from build123d import *

# Parameters (mm, degrees)
SKETCH1_R                 = 10.275
SKETCH1_R_2               = 8.275
BOSS_EXTRUDE3_DEPTH       = 5
SKETCH1_6_R               = 8.275
SKETCH1_6_R_2             = 6.025
BOSS_EXTRUDE4_DEPTH       = 18
BOSS_EXTRUDE7_DEPTH       = 40
BOSS_EXTRUDE7_DEPTH_BACK  = 70
SKETCH4_R                 = 25
SKETCH4_R_2               = 23
SKETCH7_W                 = 197.712308018
SKETCH7_H                 = 113.854833504
CUT_EXTRUDE4_DEPTH        = 64
BOSS_EXTRUDE9_START       = -2
SKETCH9_RX                = 35.355339059
SKETCH9_RY                = 25
SKETCH9_R                 = 6.025
BOSS_EXTRUDE9_DEPTH       = 2
BOSS_EXTRUDE12_DEPTH      = 2
BOSS_EXTRUDE12_DEPTH_BACK = 4
SKETCH22_W                = 69.752550136
SKETCH22_H                = 19.780641822
CUT_EXTRUDE5_DEPTH        = 10
BOSS_EXTRUDE13_START      = -2
BOSS_EXTRUDE13_DEPTH      = 2
CUT_EXTRUDE6_REACH        = 111.4
SKETCH21_R                = 2.525
CUT_EXTRUDE14_START       = -80
CUT_EXTRUDE14_DEPTH       = 80
CUT_EXTRUDE21_START       = -86
CUT_EXTRUDE21_DEPTH       = 86
SKETCH28_R                = 28.746438964
CUT_EXTRUDE22_DEPTH       = 25
CHAMFER1_SIZE             = 0.7
CHAMFER1_SIZE2            = 0.490145277


with BuildPart() as part:
    # Sketch1 → Boss-Extrude3 (new body)
    with BuildSketch(Plane(origin=(0, 0, 0), x_dir=(1, 0, 0), z_dir=(0, 1, 0))):
        with Locations(Location((0, 0, 0), (0, 0, 270))):
            Circle(SKETCH1_R)
        with Locations(Location((0, 0, 0), (0, 0, 270))):
            Circle(SKETCH1_R_2, mode=Mode.SUBTRACT)
    extrude(amount=BOSS_EXTRUDE3_DEPTH)

    # Sketch1<6> → Boss-Extrude4 (add)
    with BuildSketch(Plane(origin=(0, 0, 0), x_dir=(1, 0, 0), z_dir=(0, 1, 0))):
        with Locations(Location((0, 0, 0), (0, 0, 270))):
            Circle(SKETCH1_6_R)
        with Locations(Location((0, 0, 0), (0, 0, 270))):
            Circle(SKETCH1_6_R_2, mode=Mode.SUBTRACT)
    extrude(amount=BOSS_EXTRUDE4_DEPTH)



with BuildPart() as body_2:
    # Sketch4 → Boss-Extrude7 (new, two sides: drawn at the far end of the back side and taken through both)
    with BuildSketch(Plane(origin=(0, -5.365491749, 5.365491749), x_dir=(-1, 0, 0), z_dir=(0, 0.7071067811865458, -0.7071067811865492)).offset(-BOSS_EXTRUDE7_DEPTH_BACK)):
        with Locations(Location((0, 0, 0), (0, 0, 90))):
            Circle(SKETCH4_R)
        with Locations(Location((0, 0, 0), (0, 0, 90))):
            Circle(SKETCH4_R_2, mode=Mode.SUBTRACT)
    extrude(amount=BOSS_EXTRUDE7_DEPTH + BOSS_EXTRUDE7_DEPTH_BACK)

    # Sketch7 → Cut-Extrude4 (cut)
    with BuildSketch(Plane(origin=(0, 0, 0), x_dir=(1, 0, 0), z_dir=(0, 1, 0))):
        Rectangle(SKETCH7_W, SKETCH7_H)
    extrude(amount=CUT_EXTRUDE4_DEPTH, mode=Mode.SUBTRACT)


with BuildPart() as part_1:
    add(part.part)

    add(body_2.part)  # Boss-Extrude9 merges body 2
    # Sketch9 → Boss-Extrude9 (add)
    with BuildSketch(Plane(origin=(0, 0, 0), x_dir=(1, 0, 0), z_dir=(0, 1, 0)).offset(BOSS_EXTRUDE9_START)):
        with Locations(Location((0, 0), (0, 0, -90))):
            Ellipse(SKETCH9_RX, SKETCH9_RY)
        with Locations(Location((0, 0, 0), (0, 0, 270))):
            Circle(SKETCH9_R, mode=Mode.SUBTRACT)
    extrude(amount=BOSS_EXTRUDE9_DEPTH)

    # Sketch15 → Boss-Extrude12 (add, two sides: drawn at the far end of the back side and taken through both)
    with BuildSketch(Plane(origin=(0, -13, 0), x_dir=(1, 0, 0), z_dir=(0, 1, 0)).offset(-BOSS_EXTRUDE12_DEPTH_BACK)):
        Polygon((-18, 50.5), (-18, 5.077623205), (-11, 12.425207431), (0.436295729, 16.20866498), (9.681434559, 13.33514052), (16.664877802, 7.136081647), (20.985766733, 0), (38, 24.667240496), (38, 50.5), (31, 50.5), (31, 26.250403727), (-11, 26.250403727), (-11, 50.5), align=None)
    extrude(amount=BOSS_EXTRUDE12_DEPTH + BOSS_EXTRUDE12_DEPTH_BACK)

    # Sketch22 → Cut-Extrude5 (cut)
    with BuildSketch(Plane.XY.offset(-26.250403727)):
        Rectangle(SKETCH22_W, SKETCH22_H)
    extrude(amount=-CUT_EXTRUDE5_DEPTH, mode=Mode.SUBTRACT)

    # Boss-Extrude13: read off the stored shape, not the designer's step
    # Boss-Extrude13 outline → Boss-Extrude13 (add)
    with BuildSketch(Plane(origin=(0, 0, -26.250403727), x_dir=(-1, 0, 0), z_dir=(0, 0, -1)).offset(BOSS_EXTRUDE13_START)):
        with BuildLine():
            add(Edge.make_bspline(
                [(13.581537177, -2), (0, -16.053738297), (-13.581537177, -2)],
                knots=[2.5099124, 2.5099124, 2.5099124, 3.773272907, 3.773272907, 3.773272907], degree=2, weights=[1, 0.807036456, 1]))
            Line((13.581537177, -2), (-13.581537177, -2))
        make_face()
    extrude(amount=BOSS_EXTRUDE13_DEPTH)

    # Sketch21 → Cut-Extrude6 (cut, up to next)
    with BuildSketch(Plane(origin=(0, 0, 0), x_dir=(1, 0, 0), z_dir=(0, 1, 0)), mode=Mode.PRIVATE) as cut_extrude6_sk1:
        with Locations(Location((0, 18, 0), (0, 0, 270))):
            Circle(SKETCH21_R)
    cut_extrude6_tool1 = extrude(cut_extrude6_sk1.sketch, amount=-CUT_EXTRUDE6_REACH, mode=Mode.PRIVATE) & part_1.part
    # Sketch21 → Cut-Extrude6 (cut, up to next)
    with BuildSketch(Plane(origin=(0, 0, 0), x_dir=(1, 0, 0), z_dir=(0, 1, 0)), mode=Mode.PRIVATE) as cut_extrude6_sk2:
        with Locations(Location((15.588457268, -9, 0), (0, 0, 270))):
            Circle(SKETCH21_R)
    cut_extrude6_tool2 = extrude(cut_extrude6_sk2.sketch, amount=-CUT_EXTRUDE6_REACH, mode=Mode.PRIVATE) & part_1.part
    # Sketch21 → Cut-Extrude6 (cut, up to next)
    with BuildSketch(Plane(origin=(0, 0, 0), x_dir=(1, 0, 0), z_dir=(0, 1, 0)), mode=Mode.PRIVATE) as cut_extrude6_sk3:
        with Locations(Location((-15.588457268, -9, 0), (0, 0, 270))):
            Circle(SKETCH21_R)
    cut_extrude6_tool3 = extrude(cut_extrude6_sk3.sketch, amount=-CUT_EXTRUDE6_REACH, mode=Mode.PRIVATE) & part_1.part
    add(cut_extrude6_tool1.solids().sort_by_distance((0, 0, -18))[0], mode=Mode.SUBTRACT)
    add(cut_extrude6_tool2.solids().sort_by_distance((15.588457, 0, 9))[0], mode=Mode.SUBTRACT)
    add(cut_extrude6_tool3.solids().sort_by_distance((-15.588457, 0, 9))[0], mode=Mode.SUBTRACT)

    # Sketch25 → Cut-Extrude14 (cut)
    with BuildSketch(Plane(origin=(0, -54.862966432, 54.862966432), x_dir=(1, 0, 0), z_dir=(0, -0.7071067811865458, 0.7071067811865492)).offset(CUT_EXTRUDE14_START)):
        with BuildLine():
            Line((-18.997239916, -12.965526429), (-18.318994403, -10.280413374))
            Line((-18.318994403, -10.280413374), (-10.404229656, -15.136075873))
            Line((-10.404229656, -15.136075873), (-2.155134235, -17.219754227))
            Line((-2.155134235, -17.219754227), (4.378324516, -17.219754227))
            Line((4.378324516, -17.219754227), (10.005758959, -15.720266669))
            Line((10.005758959, -15.720266669), (15.570666352, -12.156224855))
            Line((15.570666352, -12.156224855), (20.908140469, -7.71958569))
            Line((20.908140469, -7.71958569), (21.57633395, -7.966292318))
            ThreePointArc((21.57633395, -7.966292318), (2.812653006, -22.827373547), (-18.997239916, -12.965526429))
        make_face()
    extrude(amount=CUT_EXTRUDE14_DEPTH, mode=Mode.SUBTRACT)

    # Sketch27 → Cut-Extrude21 (cut)
    with BuildSketch(Plane(origin=(0, -54.862966432, 54.862966432), x_dir=(1, 0, 0), z_dir=(0, -0.7071067811865458, 0.7071067811865492)).offset(CUT_EXTRUDE21_START)):
        with BuildLine():
            Line((-14.900346348, -17.520835559), (14.900346348, -17.520835559))
            ThreePointArc((14.900346348, -17.520835559), (0, -23), (-14.900346348, -17.520835559))
        make_face()
    extrude(amount=CUT_EXTRUDE21_DEPTH, mode=Mode.SUBTRACT)

    # Sketch28 → Cut-Extrude22 (cut)
    with BuildSketch(Plane(origin=(0, -54.862966432, 54.862966432), x_dir=(1, 0, 0), z_dir=(0, -0.7071067811865458, 0.7071067811865492))):
        Circle(SKETCH28_R)
    extrude(amount=-CUT_EXTRUDE22_DEPTH, mode=Mode.SUBTRACT)

    # Chamfer1
    chamfer1_edges = [part_1.edges().sort_by_distance(p)[0] for p in [
        (0, 18, -8.275),
    ]]
    chamfer1_side = [part_1.faces().sort_by_distance(p)[0] for p in [
        (0, 11.5, -8.275),
    ]]
    chamfer(chamfer1_edges, length=CHAMFER1_SIZE, length2=CHAMFER1_SIZE2, reference=chamfer1_side[0])


solid = part_1.part
Verification items for the finished model (mm, model axes). A direction names the side the tool comes from. Round coordinates to 2 decimals unless told otherwise and drop trailing zeros. Loops run counter-clockwise (first coordinate to the right, second up) from the corner with the lowest first, then second, coordinate; pieces in that order, holes last. Notation, with made-up numbers: (19.25, -12.75) - (59.25, -12.75) arc R28 cw to (59.25, 13.25) - close; hole circle Ø1 at (14.5, 42). An arc over 180 degrees is marked (long way). Write item = value, one per line.
Q1. Material ranges on L1, parallel to X at y = -1.05, z = 9; L2, parallel to Y at x = 5.5, z = 5; L3, parallel to Z at x = -1, y = 11, recorded low to high.
Here are the results:
L1 = -24.36 to -18.11, -13.06 to 13.06, 18.11 to 24.36
L2 = -39.49 to -36.58, -2 to 18
L3 = -8.21 to -5.94, 5.94 to 8.21
Q2. Sectioned sample at A-A on x = 0. State how many separate pieces and enclosed holes the cut face has, plus the area to 3 significant figures.
Here are the results:
separate_pieces = 3
enclosed_holes = 0
area = 415 mm^2
Q3. Mould release check, pull along Z, two halves, no side actions. Record for faces 5 (the flat face through (7.29, -52.82, 21.55)), 6 (the cylindrical face through (0.111, -0.986, -20.523)), 7 (the flat face through (5, -2, 5)), 8 (the flat face through (31, -14, -39)): +Z half, -Z half, draft (parallel to the pull), parting line (faces both ways), or undercut.
Here are the results:
face_5 = +Z half
face_6 = undercut
face_7 = undercut
face_8 = draft
Q4. Depth check by flat-ended pin: pin 1 (10 mm diameter, centred on x = 1, y = -4, fed in from -Z); pin 2 (10.5 mm diameter, centred on x = -1.5, z = 5, fed in from +Y); pin 3 (4.5 mm diameter, centred on x = 15.59, z = 9, fed in from +Y); pin 4 (12 mm diameter, centred on x = 26.5, y = -3.5, fed in from -Z). Enter the tip coordinate at first touch or a pass-through.
Here are the results:
pin_1 = -26.25
pin_2 = 18
pin_3 = -28.92
pin_4 = -19.84
Q5. Tool access check on faces 1 (the flat face through (21, -2, -18)), 2 (the flat face through (-18, -14, -29)), 3 (the cylindrical face through (-13.085, -0.986, 8.671)), 4 (the flat face through (0, -3, -26.25)). Record the directions out of +Z, -Z, +X, -X, +Y, -Y that give a thin tool (end or side, any length) a straight path to the whole face; none if there is none.
Here are the results:
face_1 = -Z, +X
face_2 = -Z, -X, -Y
face_3 = +Y
face_4 = -Z, +X, -X, +Y
Q6. Sectioned sample at B-B on x = 33. Record the boundary of the cut face in (y, z).
Here are the results:
outline = (-17, -50.5) - (-11, -50.5) - (-11, -17.42) - (-17, -17.42) - close
